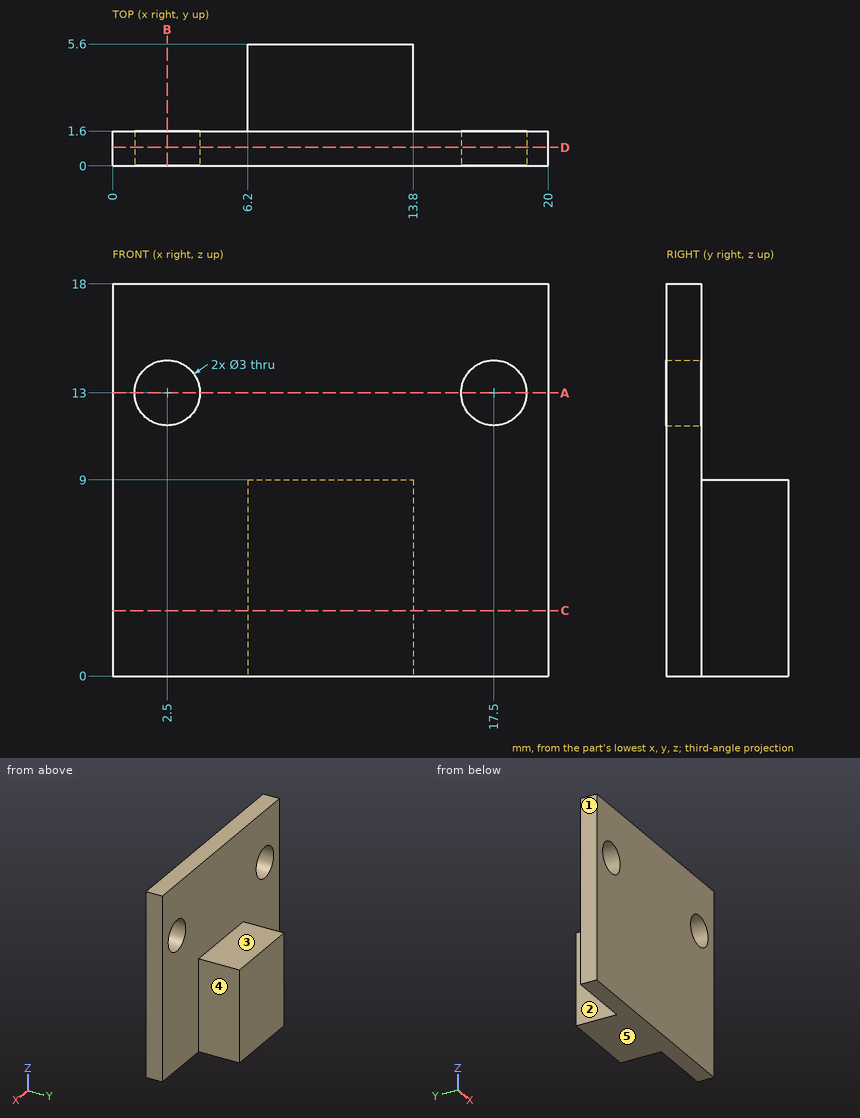
Could you check a few things on this drawing? It's one solid part, dimensions in mm from its lowest x, y, z. A direction names the side the tool comes from. Round coordinates to 2 decimals unless told otherwise and drop trailing zeros. Write each loop counter-clockwise with the first axis right and the second up, starting at its lowest first coordinate (ties: lowest second). Pieces come first, ordered by that corner, then holes.
Q1. Will these pins go through, and if not, where does the flat tip stop? P1, Ø3, axis at x = 12.5, y = 4.5, coming from the +Z side; P2, Ø3, axis at y = 3.5, z = 7, coming from the -X side; P3, Ø2, axis at y = 3, z = 4.5, coming from the +X side; P4, Ø1.8, axis at x = 2.5, z = 13, coming from the +Y side.
Q2. Please list where these lines run through material, in increasing order: probe 1 along X at (y, z) = (0.3, 13); probe 2 along Z at (x, y) = (17.5, 0.75); probe 3 along Z at (x, y) = (8.5, 2.1).
Q3. If we section it at C-C on z = 3: Write out the boundary of the cut face in (x, y).
Q4. If we section it at A-A on z = 13: Write out the boundary of the cut face in (x, y).
Q5. Which directions (+Z, -Z, +X, -X, +Y, -Y) give clear straight access to the entire face, cutting with the end or side of a thin tool? Please do the marked faces 1, 2, 3, 4 and 5.
Q6. If we section it at D-D on y = 0.85: Write out the boundary of the cut face in (x, z), plus the area to 3 significant figures.
Q7. If we section it at B-B on x = 2.5: Write out the boundary of the cut face in (y, z).
Answer below:
1. P1: stops at z = 9
1. P2: stops at x = 6.2
1. P3: stops at x = 13.8
1. P4: passes through
2. probe 1: x = 0 to 1, 4 to 16, 19 to 20
2. probe 2: z = 0 to 11.5, 14.5 to 18
2. probe 3: z = 0 to 9
3. outline: (0, 0) - (20, 0) - (20, 1.6) - (13.8, 1.6) - (13.8, 5.6) - (6.2, 5.6) - (6.2, 1.6) - (0, 1.6) - close
4. outline: (0, 0) - (1, 0) - (1, 1.6) - (0, 1.6) - close; (4, 0) - (16, 0) - (16, 1.6) - (4, 1.6) - close; (19, 0) - (20, 0) - (20, 1.6) - (19, 1.6) - close
5. face 1: +Z, -Z, -X, +Y, -Y
5. face 2: +Z, -Z, -X, +Y
5. face 3: +Z, +X, -X, +Y
5. face 4: +Z, -Z, +X, +Y
5. face 5: -Z, +X, -X, +Y, -Y
6. outline: (0, 0) - (20, 0) - (20, 18) - (0, 18) - close; hole circle Ø3 at (2.5, 13); hole circle Ø3 at (17.5, 13)
6. area: 346 mm2
7. outline: (0, 0) - (1.6, 0) - (1.6, 11.5) - (0, 11.5) - close; (0, 14.5) - (1.6, 14.5) - (1.6, 18) - (0, 18) - close
